```python
from build123d import *

# Parameters (mm, degrees)
BOSS_EXTRUDE1_DEPTH = 10
SKETCH2_R           = 11
BOSS_EXTRUDE2_DEPTH = 40
SKETCH3_R           = 6
CUT_EXTRUDE1_DEPTH  = 48.16990566
SKETCH4_R           = 2.25
CUT_EXTRUDE2_DEPTH  = 48.16990566


with BuildPart() as part:
    # Sketch1 → Boss-Extrude1 (new body)
    with BuildSketch(Plane.XY):
        with BuildLine():
            Line((-15, 13.228756555), (-15, -13.228756555))
            ThreePointArc((-15, -13.228756555), (0, -20), (15, -13.228756555))
            Line((15, -13.228756555), (15, 13.228756555))
            ThreePointArc((15, 13.228756555), (0, 20), (-15, 13.228756555))
        make_face()
    extrude(amount=BOSS_EXTRUDE1_DEPTH)

    # Sketch2 → Boss-Extrude2 (add)
    with BuildSketch(Plane(origin=(0, 0, 0), x_dir=(-1, 0, 0), z_dir=(0, 0, -1))):
        Circle(SKETCH2_R)
    extrude(amount=-BOSS_EXTRUDE2_DEPTH)

    # Sketch3 → Cut-Extrude1 (cut, through all)
    with BuildSketch(Plane.XY.offset(40)):
        Circle(SKETCH3_R)
    extrude(amount=-CUT_EXTRUDE1_DEPTH, mode=Mode.SUBTRACT)

    # Sketch4 → Cut-Extrude2 (cut, through all)
    with BuildSketch(Plane(origin=(0, 0, 0), x_dir=(-1, 0, 0), z_dir=(0, 0, -1))):
        with Locations((-11.313708499, 11.313708499)):
            Circle(SKETCH4_R)
        with Locations((0, 16)):
            Circle(SKETCH4_R)
        with Locations((11.313708499, 11.313708499)):
            Circle(SKETCH4_R)
    cut_extrude2 = extrude(amount=-CUT_EXTRUDE2_DEPTH, mode=Mode.SUBTRACT)

    # Mirror1: Cut-Extrude2 across plane
    add(cut_extrude2.mirror(Plane.ZX), mode=Mode.SUBTRACT)


solid = part.part
```
Input: part model. Units: mm. Frame: model coordinates. A direction names the side the tool comes from. Give positions to 0.01 mm unless a question says otherwise; leave off trailing zeros. Loops run counter-clockwise (first coordinate to the right, second up) from the corner with the lowest first, then second, coordinate; pieces in that order, holes last.
1) Contact query for flat-ended pins moving along their axis: pin 1 (10 mm diameter, centred on x = 11.5, z = 31.5, fed in from -Y); pin 2 (5 mm diameter, centred on y = -9.5, z = 21, fed in from -X); pin 3 (3 mm diameter, centred on x = 4.5, z = 31, fed in from -Y). Output: stop coordinate, or through.
A:
pin 1: stops at y = -8.87
pin 2: stops at x = -8.49
pin 3: stops at y = -10.58
2) Section query D-D on x = 8. Return the cut outline in (y, z), and give its area (3 significant figures).
A:
outline: (-18.33, 0) - (18.33, 0) - (18.33, 10) - (7.55, 10) - (7.55, 40) - (-7.55, 40) - (-7.55, 10) - (-18.33, 10) - close
area: 820 mm2
3) Section query C-C on y = 0. Return the cut outline in (x, z), and give its area (3 significant figures).
A:
outline: (-15, 0) - (-6, 0) - (-6, 40) - (-11, 40) - (-11, 10) - (-15, 10) - close; (6, 0) - (15, 0) - (15, 10) - (11, 10) - (11, 40) - (6, 40) - close
area: 480 mm2
4) Line query: L1, parallel to Y at x = 0.25, z = 20; L2, parallel to Y at x = -11.25, z = 9.5; L3, parallel to Z at x = 10.75, y = -4. Output: solid intervals per line, ascending.
A:
L1: y = -11 to -5.99, 5.99 to 11
L2: y = -16.54 to -13.56, -9.06 to 9.06, 13.56 to 16.54
L3: z = 0 to 10
5) Mould query, pull axis X, two halves, no side actions, for faces 1 (the flat face through (-6.5, 0.3, 0)), 2 (the cylindrical face through (2.38, -10.74, 24.79)), 3 (the cylindrical face through (-6, 0, 20)). Classes: released by +X, released by -X, zero draft, split by the parting line, or undercut.
A:
face 1: zero draft
face 2: split by the parting line
face 3: undercut
6) Reachability of faces 4 (the flat face through (-15, 0, 5)), 5 (the flat face through (-10, 5, 10)) from +Z, -Z, +X, -X, +Y, -Y: full face, straight path, thin tool, end or side. Return the list, or none.
A:
face 4: +Z, -Z, -X, +Y, -Y
face 5: +Z
7) Section query B-B on x = 0. Return the cut outline in (y, z).
A:
outline: (-20, 0) - (-18.25, 0) - (-18.25, 10) - (-20, 10) - close; (-13.75, 0) - (-6, 0) - (-6, 40) - (-11, 40) - (-11, 10) - (-13.75, 10) - close; (6, 0) - (13.75, 0) - (13.75, 10) - (11, 10) - (11, 40) - (6, 40) - close; (18.25, 0) - (20, 0) - (20, 10) - (18.25, 10) - close
8) Section query A-A on y = -16. Return the cut outline in (x, z).
A:
outline: (-12, 0) - (-2.25, 0) - (-2.25, 10) - (-12, 10) - close; (2.25, 0) - (12, 0) - (12, 10) - (2.25, 10) - close
